Verification items for the finished model (mm, model axes). A direction names the side the tool comes from. Round coordinates to 2 decimals unless told otherwise and drop trailing zeros. Write each loop counter-clockwise with the first axis right and the second up, starting at its lowest first coordinate (ties: lowest second). Pieces come first, ordered by that corner, then holes. Notation, with made-up numbers: (71, 69) - (129, 69) arc R34 ccw to (129, 108) - close; hole circle Ø8 at (-8.75, 50). An arc over 180 degrees is marked (long way). Write each question's results on one line, items separated by ' | '.
```python
from build123d import *

# Parameters (mm, degrees)
SKETCH4_R          = 3.175
CUT_EXTRUDE1_DEPTH = 12.7


with BuildPart() as part:
    # Sweep1: sweep along a path in Sketch3
    with BuildLine(Plane(origin=(0, 0, 0), x_dir=(1, 0, 0), z_dir=(0, 1, 0))) as sweep1_path:
        Line((349.25, 0), (349.25, -412.75))
        Line((349.25, -412.75), (-349.25, -412.75))
        Line((-349.25, -412.75), (-349.25, 0))
    # Sketch2 → Sweep1 (sweep)
    with BuildSketch(Plane.XY):
        with BuildLine():
            Line((-349.25, 63.5), (-393.7, 63.5))
            ThreePointArc((-393.7, 63.5), (-416.150640303, 54.200640303), (-425.45, 31.75))
            Line((-425.45, 31.75), (-425.45, -31.75))
            ThreePointArc((-425.45, -31.75), (-416.150640303, -54.200640303), (-393.7, -63.5))
            Line((-393.7, -63.5), (-349.25, -63.5))
            Line((-349.25, -63.5), (-349.25, 63.5))
        make_face()
    sweep(path=sweep1_path.line, transition=Transition.RIGHT)

    # Sketch4 → Cut-Extrude1 (cut)
    with BuildSketch(Plane(origin=(0, 0, 412.75), x_dir=(-1, 0, 0), z_dir=(0, 0, -1))):
        with Locations((-342.9, 50.8)):
            Circle(SKETCH4_R)
        with Locations((-330.2, 50.8)):
            Circle(SKETCH4_R)
        with Locations(Location((330.2, 50.8, 0), (0, 0, 180))):
            Circle(SKETCH4_R)
        with Locations(Location((342.9, 50.8, 0), (0, 0, 180))):
            Circle(SKETCH4_R)
    extrude(amount=-CUT_EXTRUDE1_DEPTH, mode=Mode.SUBTRACT)


solid = part.part
```
(1) Section check B-B (x = 280). Record the cut outline in (y, z), plus the area to 3 significant figures.
Answer:
outline: (-63.5, 412.75) - (63.5, 412.75) - (63.5, 457.2) arc R31.75 ccw to (31.75, 488.95) - (-31.75, 488.95) arc R31.75 ccw to (-63.5, 457.2) - close | area: 9,240 mm2
(2) Thickness scan on L1, parallel to Y at x = 330.2, z = 422.25 (3 decimals); L2, parallel to X at y = 35, z = 275; L3, parallel to X at y = 50, z = 419. Record the ranges inside material, lowest first.
Answer:
L1: -63.5 to 47.625, 53.975 to 63.5 | L2: -425.28 to -349.25, 349.25 to 425.28 | L3: -419.68 to -345.97, -339.83 to -333.27, -327.13 to 327.13, 333.27 to 339.83, 345.97 to 419.68
(3) Go/stop test with flat-tipped pins: pin 1 Ø7 at (x, y) = (-342, 52) entering from -Z; pin 2 Ø4 at (y, z) = (49.5, 357.5) entering from +X; pin 3 Ø5.5 at (x, y) = (-342.9, 50.8) entering from -Z. Record where each tip stops, or that it passes through.
Answer:
pin 1: z = 412.75 | pin 2: x = 421.27 | pin 3: z = 425.45
(4) Set-up check for faces 4 (the flat face through (388, 1, 0)), 5 (the flat face through (-5, -1, 412.75)): record each of +Z, -Z, +X, -X, +Y, -Y from which the full face is reachable in a straight line by a thin tool's end or side.
Answer:
face 4: -Z, +X, -X, +Y, -Y | face 5: -Z, +Y, -Y
(5) Mould release check, pull along X, two halves, no side actions. Record for faces 1 (the cylindrical face through (-416.4, 53.95, 241.05)), 2 (the flat face through (349.25, -1, 209)), 3 (the cylindrical face through (-5.96, -54.45, 479.4)): released by +X, released by -X, zero draft, split by the parting line, or undercut.
Answer:
face 1: released by -X | face 2: undercut | face 3: zero draft
(6) Section check C-C (y = -55). Record the cut outline in (x, z).
Answer:
outline: (-415.32, 0) - (-349.25, 0) - (-349.25, 412.75) - (349.25, 412.75) - (349.25, 0) - (415.32, 0) - (415.32, 478.82) - (-415.32, 478.82) - close
(7) Section check A-A (z = 50). Record the cut outline in (x, y).
Answer:
outline: (-425.45, -31.75) arc R31.75 ccw to (-393.7, -63.5) - (-349.25, -63.5) - (-349.25, 63.5) - (-393.7, 63.5) arc R31.75 ccw to (-425.45, 31.75) - close; (349.25, -63.5) - (393.7, -63.5) arc R31.75 ccw to (425.45, -31.75) - (425.45, 31.75) arc R31.75 ccw to (393.7, 63.5) - (349.25, 63.5) - close
